Autodesk Inventor part; units mm, degrees
ref_plane "YZ Plane" through (0, 0, 0) normal (1, 0, 0) x (0, 1, 0)
ref_plane "XZ Plane" through (0, 0, 0) normal (0, 1, 0) x (-1, 0, 0)
ref_plane "XY Plane" through (0, 0, 0) normal (0, 0, 1) x (1, 0, 0)
sketch "Sketch1" plane through (0, 0, 0) normal (0, 1, 0) x (-1, 0, 0)
  line L0 (0, 0) -> (0, -129.54)
  line L1 (0, 0) -> (99.06, 0)
  line L2 (99.06, 0) -> (99.06, -129.54)
  line L3 (99.06, -129.54) -> (0, -129.54)
  line L4 (140.0707, 45.2128) -> (-215.5629, 45.2128)
  line L5 (-215.5629, 45.2128) -> (-215.5629, -504.8339)
  line L6 (-215.5629, -504.8339) -> (140.0707, -504.8339)
  line L7 (140.0707, -504.8339) -> (140.0707, 45.2128)
  dimension "d0" = 129.54
  dimension "d1" = 99.06
extrude "Extrusion1" add sketch "Sketch1" against normal blind 101.6 contours L1 L2 L3 L0 | L7 L6 L5 L4
draft "FaceDraft1" angle -20 pull direction (0, -1, 0) faces at (215.5629, -33.8667, -138.1361) (-21.5262, -33.8667, 45.2128) fixed edges at (215.5629, -101.6, -229.8106) (37.7461, -101.6, 45.2128)
draft "FaceDraft2" angle -20 pull direction (0, -1, 0) faces at (-140.0707, -67.7333, -150.4626) (84.6919, -67.7333, -504.8339) fixed edges at (-140.0707, 0, -248.3003) (37.7461, -101.6, -504.8339)
sketch "Sketch2" plane through (0, 0, 0) normal (0, 1, 0) x (1, 0, 0)
  line L0 (178.5835, 467.8546) -> (215.5629, 504.8339)
  line L1 (178.5835, 467.8546) -> (79.5235, 467.8546)
  line L2 (79.5235, 467.8546) -> (79.5235, 338.3146)
  line L3 (79.5235, 338.3146) -> (178.5835, 338.3146)
  line L4 (178.5835, 338.3146) -> (178.5835, 467.8546)
  line L5 (178.5835, 338.3146) -> (178.5835, 346.4426)
  line L6 (178.5835, -8.2334) -> (178.5835, 467.8546)
  line L7 (178.5835, 467.8546) -> (178.5835, 459.7266)
  circle A0 centre (95.5255, 403.0846) radius 2.54
  circle A1 centre (169.6935, 346.4426) radius 2.54
  circle A2 centre (169.6935, 459.7266) radius 2.54
  point P0 (0, 0)
  dimension "d6" = 99.06
  dimension "d7" = 129.54
  dimension "d13" = 5.08
  dimension "d14" = 5.08
  dimension "d15" = 5.08
extrude "Extrusion2" cut sketch "Sketch2" against normal blind 5.08 contours A0 | A1 | A2
equation "\"d16\" = d14"
properties part number "Base"
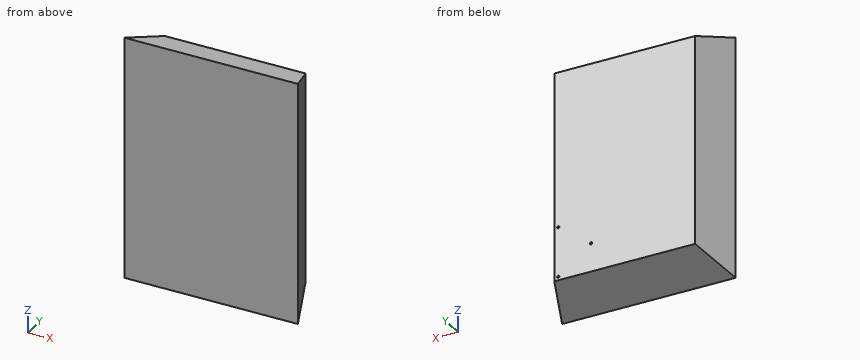
Design review of the part built by this model. Coordinates are the model's own, in mm. Give positions to 0.01 mm unless a question says otherwise; leave off trailing zeros. Order: outer loops, then holes, each group sorted by start corner. A loop starts at its lowest first (then second) coordinate and runs counter-clockwise, first axis right, second up. Notation, with made-up numbers: (6.25, 42.5) -> (40.25, 42.5) arc R20 ccw to (40.25, 46.5) -> close; hole circle Ø1 at (16, -22.75). An arc over 180 degrees is marked (long way). Write each question's results on one line, items separated by ' | '. Start each with the question number.
Q1. For pin 1 (5 mm diameter, centred on y = -67, z = -159, fed in from -X); pin 2 (8 mm diameter, centred on y = -19, z = -85.5, fed in from +X); pin 3 (8 mm diameter, centred on x = -9.5, y = -85.5, fed in from +Z), all flat-tipped, find the tip position at first contact; note any pin that passes through.
Q2. Add section B-B on x = 25. Give the boundary of the cut face in (y, z).
Q3. Wall thickness on L1, parallel to X at y = -90, z = -358.5; L2, parallel to X at y = -26.5, z = -319.5; L3, parallel to Z at x = 170.5, y = -84.5: over which ranges is each line inside the solid? List them lowest first. Write a range as from..to.
Q4. Add section A-A on z = -91.5. Give the boundary of the cut face in (x, y).
Found:
1) pin 1: stops at x = -165.37 | pin 2: stops at x = 186.95 | pin 3: stops at z = 40.81
2) outline: (-101.6, -504.83) -> (0, -467.85) -> (0, 8.23) -> (-101.6, 45.21) -> close
3) L1: x = -172.83..211.34 | L2: x = -149.72..188.23 | L3: z = -498.61..38.99
4) outline: (-177.05, -101.6) -> (215.56, -101.6) -> (178.58, 0) -> (-140.07, 0) -> close
